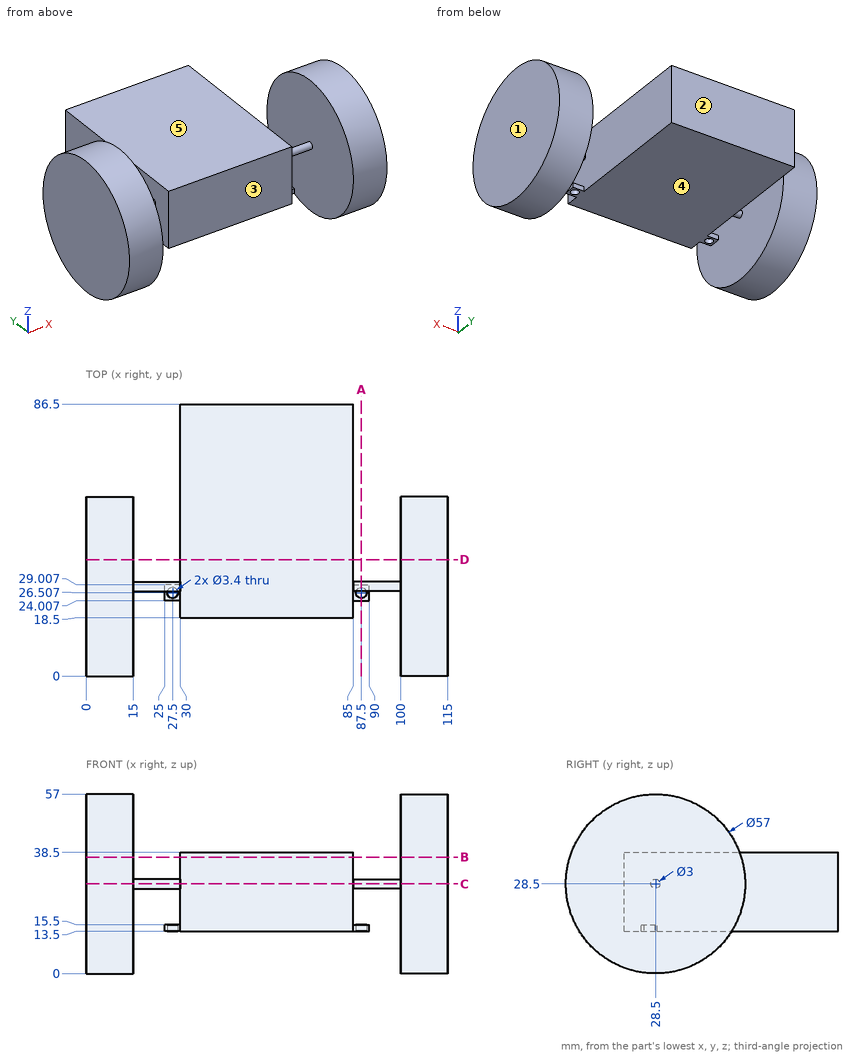
The drawing under review shows one solid part. Ordinate dimensions are in mm from its lowest x, y, z. A direction names the side the tool comes from. Coordinates: 2 decimals unless noted, no trailing zeros. Order: outer loops, then holes, each group sorted by start corner. A loop starts at its lowest first (then second) coordinate and runs counter-clockwise, first axis right, second up. Notation, with made-up numbers: (-10, 66.25) -> (-4, 66.25) arc R28 cw to (-4, 102.25) -> close; hole circle Ø6 at (44.5, -15.5). An arc over 180 degrees is marked (long way). One line per item, written item: value.
1) Clearance check with flat-ended pins moving along their axes: P1, Ø7.5, axis at y = 53, z = 27, coming from the -X side; P2, Ø0.6, axis at x = 28.5, z = 15, coming from the +Y side; P3, Ø2, axis at y = 63.5, z = 18, coming from the -X side; P4, Ø4, axis at x = 87.5, y = 26.51, coming from the +Z side. State where each tip first meets the part, or that it passes through.
Output values:
P1: stops at x = 0
P2: stops at y = 29.01
P3: stops at x = 30
P4: stops at z = 30
2) We need section C-C, the plane z = 28.5. Give the boundary of the cut face in (x, y), then the cut area to 3 significant figures.
Output values:
outline: (0, 0) -> (15, 0) -> (15, 27) -> (30, 27) -> (30, 18.5) -> (85, 18.5) -> (85, 27) -> (100, 27) -> (100, 0) -> (115, 0) -> (115, 57) -> (100, 57) -> (100, 30) -> (85, 30) -> (85, 86.5) -> (30, 86.5) -> (30, 30) -> (15, 30) -> (15, 57) -> (0, 57) -> close
area: 5,540 mm2
3) We need section D-D, the plane y = 37. Give the boundary of the cut face in (x, z), then the cut area to 3 significant figures.
Output values:
outline: (0, 1.3) -> (15, 1.3) -> (15, 55.7) -> (0, 55.7) -> close; (30, 13.5) -> (85, 13.5) -> (85, 38.5) -> (30, 38.5) -> close; (100, 1.3) -> (115, 1.3) -> (115, 55.7) -> (100, 55.7) -> close
area: 3,010 mm2
4) We need section A-A, the plane x = 87.5. Give the boundary of the cut face in (y, z).
Output values:
outline: (24.01, 13.5) -> (24.81, 13.5) -> (24.81, 15.5) -> (24.01, 15.5) -> close; circle Ø3 at (28.5, 28.5); (28.21, 13.5) -> (29.01, 13.5) -> (29.01, 15.5) -> (28.21, 15.5) -> close
5) Machinability: for the marked faces 1, 2, 3, 4 and 5, which of the approach directions +Z, -Z, +X, -X, +Y, -Y give a long, thin tool a straight path to every point of the face, cutting with its end or side? Answer none if there is none.
Output values:
face 1: +Z, -Z, +X, +Y, -Y
face 2: +Z, -Z, +X, -X, +Y
face 3: +Z, -Z, -Y
face 4: -Z, +Y, -Y
face 5: +Z, +Y, -Y
6) To check wall thickness, follow probe 1 along X at (y, z) = (43, 27); probe 2 along X at (y, z) = (53, 39); probe 3 along Y at (x, z) = (27.5, 14.9). State the ranges of each line that lie inside material, in increasing order. Write a range as [from, to].
Output values:
probe 1: x = [0, 15], [30, 85], [100, 115]
probe 2: x = [0, 15], [100, 115]
probe 3: y = [24.01, 24.81], [28.21, 29.01]
7) We need section B-B, the plane z = 37. Give the boundary of the cut face in (x, y), then the cut area to 3 significant figures.
Output values:
outline: (0, 1.3) -> (15, 1.3) -> (15, 55.7) -> (0, 55.7) -> close; (30, 18.5) -> (85, 18.5) -> (85, 86.5) -> (30, 86.5) -> close; (100, 1.3) -> (115, 1.3) -> (115, 55.7) -> (100, 55.7) -> close
area: 5,370 mm2
